from build123d import *

# Parameters (mm, degrees)
SKETCH1_R           = 49.5046
BOSS_EXTRUDE1_DEPTH = 3.175
SKETCH2_R           = 47.6885
BOSS_EXTRUDE2_DEPTH = 3.175
SKETCH3_R           = 3.175
SKETCH3_R_2         = 6.35
CUT_EXTRUDE1_DEPTH  = 7.35
CUT_EXTRUDE2_DEPTH  = 4.175


with BuildPart() as part:
    # Sketch1 → Boss-Extrude1 (new body)
    with BuildSketch(Plane.XY):
        Circle(SKETCH1_R)
    extrude(amount=BOSS_EXTRUDE1_DEPTH)

    # Sketch2 → Boss-Extrude2 (add)
    with BuildSketch(Plane.XY.offset(3.175)):
        Circle(SKETCH2_R)
    extrude(amount=BOSS_EXTRUDE2_DEPTH)

    # Sketch3 → Cut-Extrude1 (cut, through all)
    with BuildSketch(Plane.XY.offset(6.35)):
        with Locations((-31.75, 0)):
            Circle(SKETCH3_R)
        with Locations((31.75, 0)):
            Circle(SKETCH3_R)
        with Locations((-12.7, -31.235352443)):
            Circle(SKETCH3_R_2)
        with Locations((12.7, -31.235352443)):
            Circle(SKETCH3_R_2)
        with Locations((0, -36.8046)):
            Circle(SKETCH3_R)
    extrude(amount=-CUT_EXTRUDE1_DEPTH, mode=Mode.SUBTRACT)

    # Sketch4 → Cut-Extrude2 (cut, through all)
    with BuildSketch(Plane.XY.offset(3.175)):
        with BuildLine():
            Line((-50.165, 0), (-47.625, 0))
            ThreePointArc((-47.625, 0), (0, -47.625), (47.625, 0))
            Line((47.625, 0), (50.165, 0))
            ThreePointArc((50.165, 0), (0, -50.165), (-50.165, 0))
        make_face()
    extrude(amount=-CUT_EXTRUDE2_DEPTH, mode=Mode.SUBTRACT)


solid = part.part
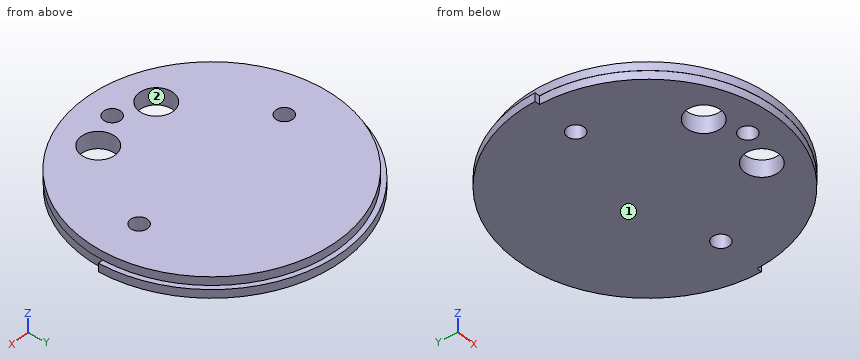
Work out the finished part from the listing and answer in its coordinate system (mm). Face numbers are marked on the shaded views. Give positions to 0.01 mm unless a question says otherwise; leave off trailing zeros. Write each loop counter-clockwise with the first axis right and the second up, starting at its lowest first coordinate (ties: lowest second). Pieces come first, ordered by that corner, then holes.
Q1. The part is cut by section C-C on x = -27. Give the vertices of the cut face in (y, z) (3 decimals), and give its area (3 significant figures).
Answer:
outline: (-39.309, 3.175) - (-39.232, 3.175) - (-39.232, 0) - (41.493, 0) - (41.493, 3.175) - (39.309, 3.175) - (39.309, 6.35) - (-39.309, 6.35) - close
area: 506 mm2
Q2. Straight lines are drawn through the part: L1, parallel to X at y = 2.5, z = 3; L2, parallel to Y at x = 0, z = 2.75 (3 decimals); L3, parallel to Z at x = -19, y = 45 (3 decimals). For each, find the intervals that lie inside material, in ascending order.
Answer:
L1: x = -49.44 to -33.71, -29.79 to 29.79, 33.71 to 49.44
L2: y = -47.625 to -39.98, -33.63 to 49.505
L3: z = 0 to 3.175
Q3. The part is cut by section A-A on x = -9. Give the vertices of the cut face in (y, z) (3 decimals).
Answer:
outline: (-46.832, 3.175) - (-46.767, 3.175) - (-46.767, 0) - (-36.396, 0) - (-36.396, 6.35) - (-46.832, 6.35) - close; (-26.075, 0) - (48.68, 0) - (48.68, 3.175) - (46.832, 3.175) - (46.832, 6.35) - (-26.075, 6.35) - close
Q4. The part is cut by section B-B on x = 31.75. Give the vertices of the cut face in (y, z) (3 decimals), and give its area (3 significant figures).
Answer:
outline: (-35.583, 3.175) - (-35.498, 3.175) - (-35.498, 0) - (-3.175, 0) - (-3.175, 6.35) - (-35.583, 6.35) - close; (3.175, 0) - (37.982, 0) - (37.982, 3.175) - (35.583, 3.175) - (35.583, 6.35) - (3.175, 6.35) - close
area: 419 mm2
Q5. Given pin 1 (1.5 mm diameter, centred on y = -18, z = 2, fed in from -X); pin 2 (1.5 mm diameter, centred on x = -48.5, z = 1.5, fed in from -Y); pin 3 (1.5 mm diameter, centred on y = -32.5, z = 2.5, fed in from -X), each flat-ended and moving along its own axis, determine where each tip first touches the part or whether it passes through.
Answer:
pin 1: stops at x = -44.39
pin 2: stops at y = 0
pin 3: stops at x = -35.5
Q6. For a pull along X with two mould halves and no side action, classify the marked faces 1 and 2 as released by +X, released by -X, zero draft, split by the parting line, or undercut.
Answer:
face 1: zero draft
face 2: undercut
